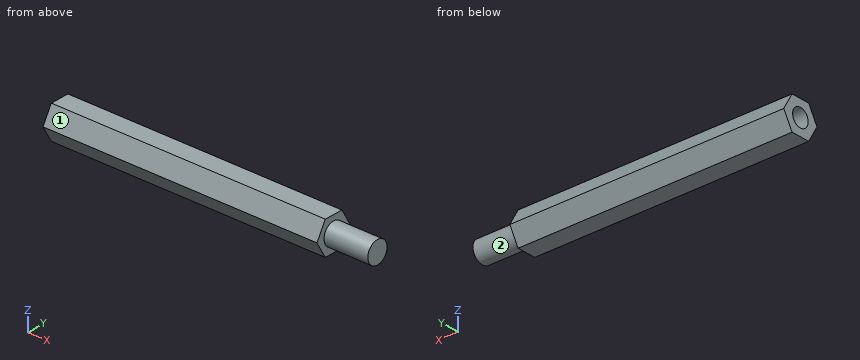
Autodesk Inventor part; units mm, degrees
ref_plane "YZ Plane" through (0, 0, 0) normal (1, 0, 0) x (0, 1, 0)
ref_plane "XZ Plane" through (0, 0, 0) normal (0, 1, 0) x (-1, 0, 0)
ref_plane "XY Plane" through (0, 0, 0) normal (0, 0, 1) x (1, 0, 0)
sketch "スケッチ1" plane through (0, 0, 0) normal (1, 0, 0) x (0, 1, 0)
  line L0 (1.7321, -3) -> (-1.7321, -3)
  line L1 (-1.7321, -3) -> (-3.4641, 0)
  line L2 (-3.4641, 0) -> (-1.7321, 3)
  line L3 (-1.7321, 3) -> (1.7321, 3)
  line L4 (1.7321, 3) -> (3.4641, 0)
  line L5 (3.4641, 0) -> (1.7321, -3)
  point P0 (0, 0)
  point P1 (0, 0)
  dimension "d0" = 6
extrude "押し出し1" add sketch "スケッチ1" along normal blind 50
sketch "スケッチ2" plane through (50, 0, 0) normal (1, 0, 0) x (0, 0, -1)
  circle A0 centre (0, 0) radius 2
  dimension "d3" = 4
extrude "押し出し2" add sketch "スケッチ2" along normal blind 8
thread "ねじ1"
sketch "スケッチ3" plane through (0, 0, 0) normal (-1, 0, 0) x (0, 0, 1)
  point P0 (0, 0)
  point P1 (0, 0)
hole "穴1" at (0, 0, 0) direction (1, 0, 0) diameter 3.242 depth 11.8 tip angle 118
properties part number "Spacer_M4_L45" material "鋼、合金"
Geometry check sheet. Reference: the model listing, model coordinates, mm. Face numbers are marked on the shaded views. A direction names the side the tool comes from. Give positions to 0.01 mm unless a question says otherwise; leave off trailing zeros. Order: outer loops, then holes, each group sorted by start corner. A loop starts at its lowest first (then second) coordinate and runs counter-clockwise, first axis right, second up. Notation, with made-up numbers: (24, 25.5) - (58, 25.5) arc R20 cw to (58, 61.5) - close; hole circle Ø1 at (-27, 9.25). An arc over 180 degrees is marked (long way). Answer as a JSON object with one key per item and string values.
(1) Cross-section at A-A (x = 33.5). Record the cut outline in (y, z).
Report:
{"outline": "(-3.46, 0) - (-1.73, -3) - (1.73, -3) - (3.46, 0) - (1.73, 3) - (-1.73, 3) - close"}
(2) Cross-section at C-C (z = 2.5). Record the cut outline in (x, y), then the cut area to 3 significant figures.
Report:
{"outline": "(0, -2.02) - (50, -2.02) - (50, 2.02) - (0, 2.02) - close", "area": "202 mm^2"}
(3) Material ranges on line 1 (Y direction, x = 8, z = 0); line 2 (Z direction, x = 3.75, y = 0); line 3 (Y direction, x = 9, z = -0.85), recorded low to high.
Report:
{"line 1": "-3.46 to -1.62, 1.62 to 3.46", "line 2": "-3 to -1.62, 1.62 to 3", "line 3": "-2.97 to -1.38, 1.38 to 2.97"}
(4) Cross-section at B-B (x = 50.5). Record the cut outline in (y, z).
Report:
{"outline": "circle Ø4 at (0, 0)"}
(5) Tool access check on the marked faces 1 and 2. Record the directions out of +Z, -Z, +X, -X, +Y, -Y that give a thin tool (end or side, any length) a straight path to the whole face; none if there is none.
Report:
{"face 1": "+Z, +X, -X, -Y", "face 2": "+X"}
